Build history of the part. All positions in model axes, mm. Face numbers are marked on the shaded views. A direction names the side the tool comes from. Round coordinates to 2 decimals unless told otherwise and drop trailing zeros. Write each loop counter-clockwise with the first axis right and the second up, starting at its lowest first coordinate (ties: lowest second). Pieces come first, ordered by that corner, then holes.
1) Saw through at A-A (z = 0). Write the cut outline in (x, y).
2) Saw through at D-D (z = -4). Write the cut outline in (x, y), plus the area to 3 significant figures.
3) Which spindle directions (+Z, -Z, +X, -X, +Y, -Y) get a long thin tool onto all of the face, cutting with end or side? Do the marked faces 1 and 2. Say none if no direction does.
4) Wall check: probe 1 along Y at (x, z) = (-3.25, -1.5); probe 2 along Z at (x, y) = (0, -15); probe 3 along X at (y, z) = (-7.5, -2). Give the ranges that are in metal, low to high.
5) Saw through at C-C (y = 2.5). Write the cut outline in (x, z).
6) Saw through at B-B (x = 0). Write the cut outline in (y, z).
7) Flat gauge pins, fed straight in: pin 1 (1.5 mm diameter, centred on y = -15.5, z = -0.5, fed in from -X); pin 2 (1.5 mm diameter, centred on y = -7, z = -3, fed in from +X); pin 3 (1.5 mm diameter, centred on x = 0.5, y = -15.5, fed in from +Z); pin 4 (3 mm diameter, centred on x = -2.5, z = 2, fed in from -Y). Where does each tip first touch, or does it go through?
from build123d import *

# Parameters (mm, degrees)
SKETCH1_R           = 5
BOSS_EXTRUDE1_DEPTH = 6
SKETCH2_R           = 3
BOSS_EXTRUDE2_DEPTH = 25
CHAMFER1_SIZE       = 1


with BuildPart() as part:
    # Sketch1 → Boss-Extrude1 (new body)
    with BuildSketch(Plane(origin=(0, 0, 0), x_dir=(1, 0, 0), z_dir=(0, 1, 0))):
        Circle(SKETCH1_R)
    extrude(amount=BOSS_EXTRUDE1_DEPTH)

    # Sketch2 → Boss-Extrude2 (add)
    with BuildSketch(Plane.XZ):
        Circle(SKETCH2_R)
    extrude(amount=BOSS_EXTRUDE2_DEPTH)

    # Chamfer1
    chamfer1_edges = [part.edges().sort_by_distance(p)[0] for p in [
        (-3, -25, 0),
    ]]
    chamfer(chamfer1_edges, length=CHAMFER1_SIZE)


solid = part.part
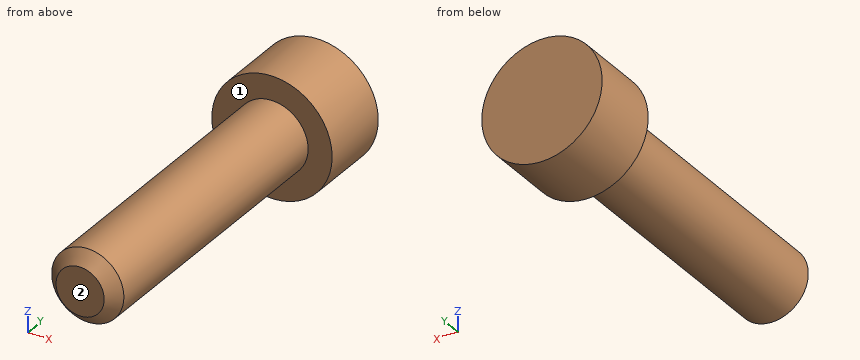
Evaluation:
1. outline: (-5, 0) - (-3, 0) - (-3, -24) - (-2, -25) - (2, -25) - (3, -24) - (3, 0) - (5, 0) - (5, 6) - (-5, 6) - close
2. outline: (-3, 0) - (3, 0) - (3, 6) - (-3, 6) - close
2. area: 36.0 mm2
3. face 1: -Y
3. face 2: +Z, -Z, +X, -X, -Y
4. probe 1: y = 0 to 6
4. probe 2: z = -3 to 3
4. probe 3: x = -2.24 to 2.24
5. outline: circle Ø10 at (0, 0)
6. outline: (-25, -2) - (-24, -3) - (0, -3) - (0, -5) - (6, -5) - (6, 5) - (0, 5) - (0, 3) - (-24, 3) - (-25, 2) - close
7. pin 1: stops at x = -3
7. pin 2: stops at x = 1.98
7. pin 3: stops at z = 3
7. pin 4: stops at y = -25
